The listing builds one solid part. Answer for the finished solid, in the listing's coordinates (mm). Face numbers are marked on the shaded views. A direction names the side the tool comes from. Give positions to 0.01 mm unless a question says otherwise; leave off trailing zeros. Loops run counter-clockwise (first coordinate to the right, second up) from the corner with the lowest first, then second, coordinate; pieces in that order, holes last. Notation, with made-up numbers: (62.5, -37.75) - (71.5, -37.75) arc R27 cw to (71.5, -12.75) - close; hole circle Ø2 at (71.25, 23). An arc over 180 degrees is marked (long way). Write item = value, one per line. Start each with the question number.
1) Consider probe 1 along Y at (x, z) = (27.75, -15) (3 decimals); probe 2 along Z at (x, y) = (27.25, 6.56); probe 3 along X at (y, z) = (59.5, -19). Determine where each line is inside the solid, lowest interval first.
2) The part is cut by section D-D on x = 32. Write down the section's boundary in (y, z), plus the area to 3 significant figures.
3) Flat-ended cylindrical pins translate along their axes: P1, Ø1, axis at y = 74, z = -3.5, coming from the +X side; P2, Ø10, axis at y = 5.5, z = -12, coming from the -X side; P3, Ø8, axis at y = 80, z = -3.5, coming from the +X side; P4, Ø3, axis at y = 23.56, z = -15, coming from the -X side. Find the tip coordinate at first contact, or state that the pin passes through.
4) Which of the six approach directions +Z, -Z, +X, -X, +Y, -Y give full straight-line access (tool end or side, diameter ignored) to the marked faces 1, 2 and 3?
5) The part is cut by section A-A on y = 23.56. Write down the section's boundary in (x, z).
6) The part is cut by section C-C on y = 76.5. Write down the section's boundary in (x, z), plus the area to 4 significant figures.
7) The part is cut by section B-B on z = -15. State how many separate pieces and enclosed holes the cut face has, plus the area to 3 significant figures.
8) The mould has two halves that part along Y. Classify the marked faces 4, 5, 6 and 7: +Y half, -Y half, draft (parallel to the pull), parting line (faces both ways), or undercut.
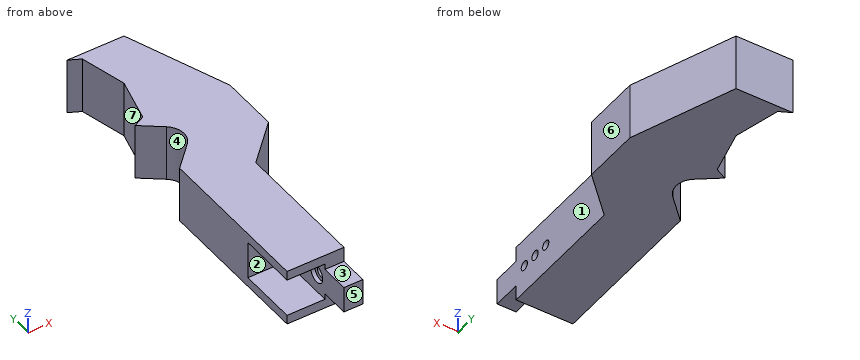
Autodesk Inventor part; units mm, degrees
ref_plane "YZ Plane" through (0, 0, 0) normal (1, 0, 0) x (0, 1, 0)
ref_plane "XZ Plane" through (0, 0, 0) normal (0, 1, 0) x (-1, 0, 0)
ref_plane "XY Plane" through (0, 0, 0) normal (0, 0, 1) x (1, 0, 0)
sketch "Sketch1" plane through (0, 0, 0) normal (0, 0, 1) x (1, 0, 0)
  line L0 (0, 0) -> (25, 0)
  line L1 (25, 0) -> (25, 40)
  line L2 (25, 40) -> (0, 40)
  line L3 (0, 40) -> (0, 0)
  dimension "d1" = 25
  dimension "d2" = 40
  dimension "d3" = 25
extrude "Extrusion1" add sketch "Sketch1" against normal blind 30
sketch "Sketch2" plane through (25, 0, 0) normal (1, 0, 0) x (0, 0, -1)
  line L0 (0, 0) -> (30, 0)
  circle A0 centre (15, 6.56) radius 2.46
extrude "Extrusion2" cut sketch "Sketch2" against normal blind 30
sketch "Sketch3" plane through (0, 0, 0) normal (-1, 0, 0) x (0, 0, 1)
  line L0 (0, 0) -> (-30, 0)
  line L1 (-25.05, 0) -> (-4.95, 0)
  line L2 (-4.95, 0) -> (-4.95, 33.12)
  line L3 (-4.95, 33.12) -> (-25.05, 33.12)
  line L4 (-25.05, 33.12) -> (-25.05, 0)
  dimension "d11" = 20.1
extrude "Extrusion3" cut sketch "Sketch3" against normal blind 20
sketch "Sketch4" plane through (0, 0, 0) normal (0, -1, 0) x (1, 0, 0)
  line L0 (20, -4.95) -> (20, -25.05)
  line L1 (20, -15) -> (25, -15)
  line L2 (25, 0) -> (25, -30)
  line L3 (20, -8.025) -> (25, -8.025)
  line L4 (25, -8.025) -> (25, -21.975)
  line L5 (25, -21.975) -> (20, -21.975)
  line L6 (20, -21.975) -> (20, -8.025)
  line L7 (20, -8.025) -> (25, -21.975) construction
  line L8 (25, -8.025) -> (20, -21.975) construction
  line L9 (25, -12.54) -> (25, -17.46)
  point P0 (0, 0)
  point P1 (22.5, -15)
  dimension "d14" = 13.95
extrude "Extrusion4" add sketch "Sketch4" along normal blind 15
sketch "Sketch5" plane through (20, 0, 0) normal (-1, 0, 0) x (0, 0, 1)
  circle A0 centre (-15, 6.56) radius 2.46
  circle A1 centre (-15, 6.56) radius 4.7025
  circle A2 centre (-15, 6.56) radius 2.46
  circle A3 centre (-15, 6.56) radius 2.46
  point P0 (0, 0)
  dimension "d17" = 9.405
extrude "Extrusion5" cut sketch "Sketch5" against normal blind 2.1
sketch "Sketch6" plane through (25, 0, 0) normal (1, 0, 0) x (0, 0, -1)
  circle A0 centre (15, 6.56) radius 4.7025
  line L0 (15, 6.56) -> (15, 23.56)
  circle A1 centre (15, 23.56) radius 2.46
  point P0 (0, 0)
  dimension "d20" = 17
  dimension "d21" = 4.92
extrude "Extrusion6" cut sketch "Sketch6" against normal blind 10 contours A1
sketch "Sketch7" plane through (20, 0, 0) normal (-1, 0, 0) x (0, 0, 1)
  circle A0 centre (-15, 23.56) radius 2.46
  circle A1 centre (-15, 23.56) radius 4.7025
  point P0 (0, 0)
  dimension "d24" = 9.405
extrude "Extrusion7" cut sketch "Sketch7" against normal blind 2.1
sketch "Sketch9" plane through (25, 0, 0) normal (1, 0, 0) x (0, 0, -1)
  circle A0 centre (15, 6.56) radius 2.46
  circle A1 centre (15, 6.56) radius 2.46
  circle A2 centre (15, 23.56) radius 2.46
  circle A3 centre (15, 23.56) radius 2.46
  line L0 (30, 40) -> (30, 0)
  line L1 (30, 0) -> (30, 40)
  line L2 (30, 40) -> (0, 40)
  line L3 (0, 40) -> (0, 0)
  line L4 (0, 0) -> (8.025, 0)
  line L5 (21.975, 0) -> (21.975, -15)
  line L6 (21.975, -15) -> (8.025, -15)
  line L7 (8.025, -15) -> (8.025, 0)
  line L8 (0, 0) -> (8.025, 0)
  line L9 (21.975, 0) -> (30, 0)
extrude "Extrusion8" add sketch "Sketch9" along normal blind 5
sketch "Sketch10" plane through (0, 40, 0) normal (0, 1, 0) x (1, 0, 0)
  line L0 (0, 30) -> (30, 30)
  line L1 (30, 0) -> (0, 0)
  line L2 (0, 30) -> (30, 30)
  line L3 (30, 30) -> (30, 0)
  line L4 (30, 0) -> (0, 0)
  line L5 (0, 0) -> (0, 30)
extrude "Extrusion9" add sketch "Sketch10" along normal blind 30
sketch "Sketch12" plane through (30, 0, 0) normal (1, 0, 0) x (0, 0, -1)
  circle A0 centre (15, 6.56) radius 2.46
  line L0 (15, 6.56) -> (15, 15.06)
  circle A1 centre (15, 15.06) radius 2.525
  point P0 (0, 0)
  dimension "d31" = 8.5
  dimension "d33" = 5.05
extrude "Extrusion10" cut sketch "Sketch12" against normal blind 30 contours A1
sketch "Sketch15" plane through (0, 0, -25.05) normal (-1, 0, 0) x (0, 0, 1)
  line L0 (0, 33.12) -> (20.1, 33.12)
  line L1 (20.1, 33.12) -> (20.1, 0)
  line L2 (0, 33.12) -> (20.1, 33.12)
  line L3 (20.1, 33.12) -> (20.1, 31.1)
  line L4 (20.1, 31.1) -> (0, 31.1)
  line L5 (0, 31.1) -> (0, 33.12)
  point P0 (25.05, 0)
  dimension "d57" = 2.02
extrude "Extrusion13" add sketch "Sketch15" against normal blind 20
sketch "Sketch17" plane through (0, 0, 0) normal (0, 0, 1) x (1, 0, 0)
  line L0 (0, 70) -> (30, 70)
  line L1 (30, 70) -> (50.0622, 90.0622)
  line L2 (30, 70) -> (80, 70) construction
  line L3 (11.9522, 97.2454) -> (0, 85.2932)
  line L4 (0, 70) -> (0, 85.2932)
  line L5 (0, 70) -> (0, 0)
  line L6 (0, 70) -> (30, 70)
  line L7 (10.923, 112.2849) -> (0, 120.567)
  line L8 (50.0622, 105.3553) -> (50.0622, 120.567)
  line L9 (50.0622, 105.3553) -> (50.0622, 90.0622)
  arc A0 (11.9522, 97.2454) -> (10.923, 112.2849) centre (4.8811, 104.3165) ccw
  line L10 (0, 174.567) -> (30, 174.567)
  line L11 (30, 174.567) -> (50.0622, 120.567)
  line L12 (6, 171.567) -> (0, 174.567)
  line L13 (6, 123.567) -> (0, 120.567)
  line L14 (6, 123.567) -> (12, 147.567)
  line L15 (6, 171.567) -> (12, 147.567)
  dimension "d61" = 45
  dimension "d62" = 32.0271
  dimension "d72" = 10
extrude "Extrusion14" add sketch "Sketch17" against normal blind 30
properties part number "rec_c_48mm_x_30mm"
Answer below:
q1.probe_1 = -15 to 4.1, 9.02 to 12.535, 17.585 to 21.1, 26.02 to 174.567
q1.probe_2 = -30 to -17.46, -12.54 to 0
q1.probe_3 = 0 to 30
q2.outline = (72, -30) - (169.18, -30) - (169.18, 0) - (72, 0) - close
q2.area = 2,920 mm2
q3.P1 = 34.5
q3.P2 = 20
q3.P3 = 44
q3.P4 = through
q4.face_1 = +Z, -Z, +X, -Y
q4.face_2 = -X, -Y
q4.face_3 = +Z, +X, -X, -Y
q5.outline = (0, -30) - (30, -30) - (30, -17.46) - (22.1, -17.46) - (22.1, -19.7) - (20, -19.7) - (20, -25.05) - (0, -25.05) - close; (0, -4.95) - (20, -4.95) - (20, -10.3) - (22.1, -10.3) - (22.1, -12.54) - (30, -12.54) - (30, 0) - (0, 0) - close
q6.outline = (0, -30) - (36.5, -30) - (36.5, 0) - (0, 0) - close
q6.area = 1,095 mm2
q7.separate_pieces = 4
q7.enclosed_holes = 0
q7.area = 5,180 mm2
q8.face_4 = undercut
q8.face_5 = -Y half
q8.face_6 = draft
q8.face_7 = undercut
